from build123d import *

# Parameters (mm, degrees)
SKETCH1_W            = 110
SKETCH1_H            = 60
BOSS_EXTRUDE1_DEPTH  = 10
SKETCH3_W            = 93.6
SKETCH3_H            = 43.6
BOSS_EXTRUDE2_DEPTH  = 7
SKETCH4_W            = 22.2
SKETCH4_H            = 24.2
CUT_EXTRUDE1_DEPTH   = 7
FILLET1_R            = 11.8
FILLET1_OF_MIRROR1_R = 11.8


with BuildPart() as part:
    # Sketch1 → Boss-Extrude1 (new body)
    with BuildSketch(Plane.XY):
        with Locations((55, 30)):
            Rectangle(SKETCH1_W, SKETCH1_H)
    extrude(amount=BOSS_EXTRUDE1_DEPTH)

    # Sketch3 → Boss-Extrude2 (add)
    with BuildSketch(Plane.XY.offset(10)):
        with Locations((55, 30)):
            Rectangle(SKETCH3_W, SKETCH3_H)
    extrude(amount=BOSS_EXTRUDE2_DEPTH)

    # Sketch4 → Cut-Extrude1 (cut)
    with BuildSketch(Plane.XY.offset(17)):
        with Locations((37.1, 20.3)):
            Rectangle(SKETCH4_W, SKETCH4_H)
    cut_extrude1 = extrude(amount=-CUT_EXTRUDE1_DEPTH, mode=Mode.SUBTRACT)

    # Fillet1
    fillet1_edges = [part.edges().sort_by_distance(p)[0] for p in [
        (26, 32.4, 13.5),
    ]]
    fillet(fillet1_edges, radius=FILLET1_R)

    # Mirror1: Cut-Extrude1 across plane
    add(cut_extrude1.mirror(Plane.ZY.offset(-55)), mode=Mode.SUBTRACT)

    # Fillet1 of Mirror1
    fillet1_of_mirror1_edges = [part.edges().sort_by_distance(p)[0] for p in [
        (84, 32.4, 13.5),
    ]]
    fillet(fillet1_of_mirror1_edges, radius=FILLET1_OF_MIRROR1_R)


solid = part.part
Work out the finished part from the listing and answer in its coordinate system (mm). A direction names the side the tool comes from. Give positions to 0.01 mm unless a question says otherwise; leave off trailing zeros. Write each loop counter-clockwise with the first axis right and the second up, starting at its lowest first coordinate (ties: lowest second). Pieces come first, ordered by that corner, then holes. Notation, with made-up numbers: (28, 87.5) - (36, 87.5) arc R24 ccw to (36, 112.5) - close; hole circle Ø3 at (-4, -23). An arc over 180 degrees is marked (long way). One line per item, written item: value. Start each with the question number.
1. Find section C-C (y = 35.5). Write down the section's boundary in (x, z).
2. Consider probe 1 along X at (y, z) = (12.5, 12.75); probe 2 along X at (y, z) = (29.5, 12); probe 3 along Z at (x, y) = (6.5, 18.5). Determine where each line is inside the solid, lowest interval first.
3. For a pull along X with two mould halves and no side action, classify faces 4 (the flat face through (66, 24, 10)), 5 (the flat face through (54, 51.8, 13)), 6 (the flat face through (110, 30, 5)) as +X half, -X half, draft (parallel to the pull), parting line (faces both ways), or undercut.
4. Find section B-B (x = 45). Write down the section's boundary in (y, z).
5. Find section A-A (z = 14.75). Write down the section's boundary in (x, y), then the cut area to 3 significant figures.
6. Given pin 1 (3.5 mm diameter, centred on x = 44.5, z = 12, fed in from +Y); pin 2 (3.5 mm diameter, centred on x = 92.5, z = 13, fed in from -Y); pin 3 (2 mm diameter, centred on y = 40, z = 14.5, fed in from -X), each flat-ended and moving along its own axis, determine where each tip first touches the part or whether it passes through.
7. For faces 1 (the flat face through (8.2, 30, 13)), 2 (the flat face through (67, 32.4, 14)), 3 (the flat face through (17, 8.2, 13)), determine the directions among +Z, -Z, +X, -X, +Y, -Y from which every point of the face is accessible in a straight line to the end or side of a thin tool.
8. Find section D-D (y = 25.5). Write down the section's boundary in (x, z).
Geometry results:
1. outline: (0, 0) - (110, 0) - (110, 10) - (101.8, 10) - (101.8, 17) - (8.2, 17) - (8.2, 10) - (0, 10) - close
2. probe 1: 8.2 to 26, 48.2 to 61.8, 84 to 101.8
2. probe 2: 8.2 to 30.05, 48.2 to 61.8, 79.95 to 101.8
2. probe 3: 0 to 10
3. face 4: undercut
3. face 5: draft
3. face 6: +X half
4. outline: (0, 0) - (60, 0) - (60, 10) - (51.8, 10) - (51.8, 17) - (32.4, 17) - (32.4, 10) - (0, 10) - close
5. outline: (8.2, 8.2) - (26, 8.2) - (26, 20.6) arc R11.8 cw to (37.8, 32.4) - (48.2, 32.4) - (48.2, 8.2) - (61.8, 8.2) - (61.8, 32.4) - (72.2, 32.4) arc R11.8 cw to (84, 20.6) - (84, 8.2) - (101.8, 8.2) - (101.8, 51.8) - (8.2, 51.8) - close
5. area: 3,070 mm2
6. pin 1: y = 51.8
6. pin 2: y = 8.2
6. pin 3: x = 8.2
7. face 1: +Z, -X, +Y, -Y
7. face 2: +Z, -Y
7. face 3: +Z, +X, -X, -Y
8. outline: (0, 0) - (110, 0) - (110, 10) - (101.8, 10) - (101.8, 17) - (82.93, 17) - (82.93, 10) - (61.8, 10) - (61.8, 17) - (48.2, 17) - (48.2, 10) - (27.07, 10) - (27.07, 17) - (8.2, 17) - (8.2, 10) - (0, 10) - close
